Design review of the part built by this model. Coordinates are the model's own, in mm. Face numbers are marked on the shaded views. A direction names the side the tool comes from. Give positions to 0.01 mm unless a question says otherwise; leave off trailing zeros. Write each loop counter-clockwise with the first axis right and the second up, starting at its lowest first coordinate (ties: lowest second). Pieces come first, ordered by that corner, then holes. Notation, with made-up numbers: (-6, -15.5) -> (12, -15.5) arc R31 ccw to (12, 19.5) -> close; hole circle Ø5 at (-11, 32). An arc over 180 degrees is marked (long way). Return JSON: item names as keys, results as strings. Group by question number.
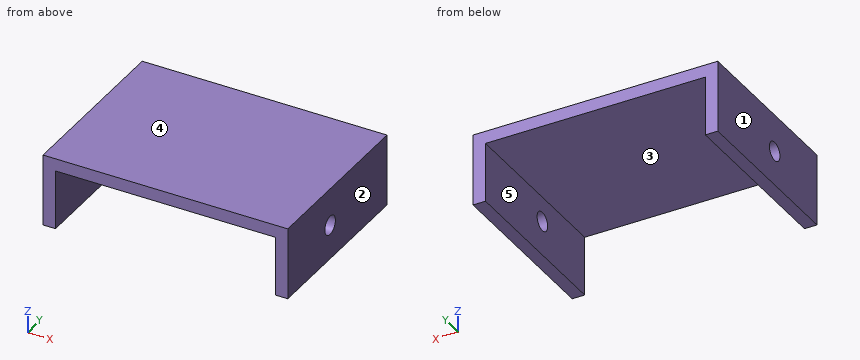
from build123d import *

# Parameters (mm, degrees)
SKETCH1_W           = 35.2
SKETCH1_H           = 28.13
BOSS_EXTRUDE1_DEPTH = 2
SKETCH2_W           = 11.528235963
SKETCH2_H           = 28.13
BOSS_EXTRUDE2_DEPTH = 2
SKETCH3_W           = 11.528235963
SKETCH3_H           = 28.13
BOSS_EXTRUDE3_DEPTH = 2
SKETCH4_R           = 1.5
CUT_EXTRUDE1_DEPTH  = 43.722962275


with BuildPart() as part:
    # Sketch1 → Boss-Extrude1 (new body)
    with BuildSketch(Plane.XY):
        Rectangle(SKETCH1_W, SKETCH1_H)
    extrude(amount=BOSS_EXTRUDE1_DEPTH)

    # Sketch2 → Boss-Extrude2 (add)
    with BuildSketch(Plane(origin=(17.6, 0, 0), x_dir=(0, 0, -1), z_dir=(1, 0, 0))):
        with Locations((3.764117982, 0)):
            Rectangle(SKETCH2_W, SKETCH2_H)
    extrude(amount=BOSS_EXTRUDE2_DEPTH)

    # Sketch3 → Boss-Extrude3 (add)
    with BuildSketch(Plane.ZY.offset(17.6)):
        with Locations((-3.764117982, 0)):
            Rectangle(SKETCH3_W, SKETCH3_H)
    extrude(amount=BOSS_EXTRUDE3_DEPTH)

    # Sketch4 → Cut-Extrude1 (cut, through all)
    with BuildSketch(Plane(origin=(19.6, 0, 0), x_dir=(0, 0, -1), z_dir=(1, 0, 0))):
        with Locations((4, -2.065)):
            Circle(SKETCH4_R)
    extrude(amount=-CUT_EXTRUDE1_DEPTH, mode=Mode.SUBTRACT)


solid = part.part
Q1. Tool access review of the marked faces 4 and 5: name each direction out of +Z, -Z, +X, -X, +Y, -Y from which nothing blocks a thin tool from reaching the whole face with its end or side.
Q2. For L1, parallel to X at y = -7.25, z = -1; L2, parallel to Y at x = -18.7, z = -4 (3 decimals); L3, parallel to Z at x = -4.5, y = -7.5, list the stretches that pass through material, from the lowest coordinate up. Write a range as from..to.
Q3. Insertion check: pin 1 (8.5 mm diameter, centred on x = -1, y = -6.5, fed in from -Z). The pin has a flat end and moves straight along its axis. Give the tip position at first contact, or say it passes through.
Q4. Take a section at D-D, the plane x = -2. Give the boundary of the cut face in (y, z) (3 decimals).
Q5. Take a section at B-B, the plane z = -0.75. Give the boundary of the cut face in (x, y) (3 decimals), plus the area to 3 significant figures.
Q6. Take a section at A-A, the plane z = -4. Give the boundary of the cut face in (x, y) (3 decimals).
Q7. Mouldability with a two-part tool opening along X and no side actions: class the marked faces 1, 2 and 3 as +X half, -X half, draft (parallel to the pull), parting line (faces both ways), or undercut.
Q8. Take a section at C-C, the plane y = 9. Give the boundary of the cut face in (x, z), plus the area to 3 significant figures.
Final values:
{
 "1": {"face 4": "+Z, +X, -X, +Y, -Y", "face 5": "-Z, +Y, -Y"},
 "2": {"L1": "x = -19.6..-17.6, 17.6..19.6", "L2": "y = -14.065..-3.565, -0.565..14.065", "L3": "z = 0..2"},
 "3": {"pin 1": "stops at z = 0"},
 "4": {"outline": "(-14.065, 0) -> (14.065, 0) -> (14.065, 2) -> (-14.065, 2) -> close"},
 "5": {"outline": "(-19.6, -14.065) -> (-17.6, -14.065) -> (-17.6, 14.065) -> (-19.6, 14.065) -> close; (17.6, -14.065) -> (19.6, -14.065) -> (19.6, 14.065) -> (17.6, 14.065) -> close", "area": "113 mm²"},
 "6": {"outline": "(-19.6, -14.065) -> (-17.6, -14.065) -> (-17.6, -3.565) -> (-19.6, -3.565) -> close; (-19.6, -0.565) -> (-17.6, -0.565) -> (-17.6, 14.065) -> (-19.6, 14.065) -> close; (17.6, -14.065) -> (19.6, -14.065) -> (19.6, -3.565) -> (17.6, -3.565) -> close; (17.6, -0.565) -> (19.6, -0.565) -> (19.6, 14.065) -> (17.6, 14.065) -> close"},
 "7": {"face 1": "-X half", "face 2": "+X half", "face 3": "undercut"},
 "8": {"outline": "(-19.6, -9.53) -> (-17.6, -9.53) -> (-17.6, 0) -> (17.6, 0) -> (17.6, -9.53) -> (19.6, -9.53) -> (19.6, 2) -> (-19.6, 2) -> close", "area": "117 mm²"}
}
